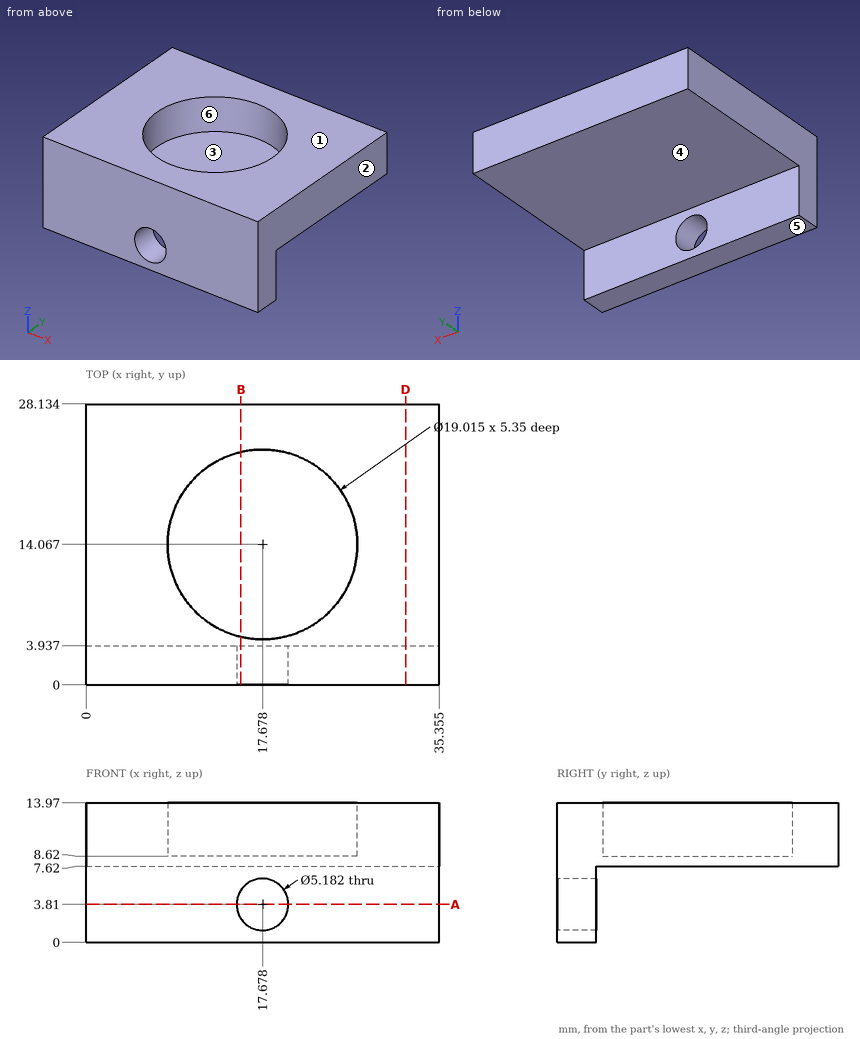
For this review, use the dimensioned drawing (mm, ordinates from the lowest corner) and the shaded views. A direction names the side the tool comes from. Coordinates: 2 decimals unless noted, no trailing zeros. Loops run counter-clockwise (first coordinate to the right, second up) from the corner with the lowest first, then second, coordinate; pieces in that order, holes last. Notation, with made-up numbers: (-22.75, -35) - (-16.75, -35) arc R24 ccw to (-16.75, -13) - close; hole circle Ø1 at (-18, -18). An arc over 180 degrees is marked (long way). Use CSV: the item, a comma, the result in double quotes. Start each with the question number.
1) Consider section B-B on x = 15.5. Write out the cut boundary in (y, z).
2) The part is to be moulded in two halves that separate along X. For the marked faces 1, 2 and 3, say which applies: +X half, -X half, draft (parallel to the pull), parting line (faces both ways), or undercut.
3) Tool access review of the marked faces 4, 5 and 6: name each direction out of +Z, -Z, +X, -X, +Y, -Y from which nothing blocks a thin tool from reaching the whole face with its end or side.
4) Consider section D-D on x = 32. Write out the cut boundary in (y, z), then the cut area to 3 significant figures.
5) For pin 1 Ø6 at (x, z) = (17.68, 3.81) entering from +Y; pin 2 Ø9.5 at (x, y) = (19, 18) entering from +Z; pin 3 Ø6 at (x, y) = (14.5, 13) entering from -Z, all flat-tipped, find the tip position at first contact; note any pin that passes through.
6) Consider section A-A on z = 3.81. Write out the cut boundary in (x, y) (1 decimal), then the cut area to 3 significant figures.
7) Wall thickness on L1, parallel to Z at x = 26, y = 18.75; L2, parallel to Y at x = 20, z = 13 (1 decimal); L3, parallel to Y at x = 10.5, z = 4.25: over which ranges is each line inside the solid? List them lowest first. Write a range as from..to.
Geometry says:
1,outline,"(0, 0) - (3.94, 0) - (3.94, 2.41) - (0, 2.41) - close; (0, 5.21) - (3.94, 5.21) - (3.94, 7.62) - (28.13, 7.62) - (28.13, 13.97) - (23.32, 13.97) - (23.32, 8.62) - (4.81, 8.62) - (4.81, 13.97) - (0, 13.97) - close"
2,face 1,"draft"
2,face 2,"+X half"
2,face 3,"undercut"
3,face 4,"-Z, +X, -X, +Y"
3,face 5,"-Z, +X, -X, +Y, -Y"
3,face 6,"+Z"
4,outline,"(0, 0) - (3.94, 0) - (3.94, 7.62) - (28.13, 7.62) - (28.13, 13.97) - (0, 13.97) - close"
4,area,"209 mm^2"
5,pin 1,"y = 3.94"
5,pin 2,"z = 8.62"
5,pin 3,"z = 7.62"
6,outline,"(0, 0) - (15.1, 0) - (15.1, 3.9) - (0, 3.9) - close; (20.3, 0) - (35.4, 0) - (35.4, 3.9) - (20.3, 3.9) - close"
6,area,"119 mm^2"
7,L1,"7.62..13.97"
7,L2,"0..4.8, 23.3..28.1"
7,L3,"0..3.94"
